Source: CAD feature listing. Evaluate the final solid. Frame: model axes, mm. Coordinates: 2 decimals unless noted, no trailing zeros. Loops run counter-clockwise (first coordinate to the right, second up) from the corner with the lowest first, then second, coordinate; pieces in that order, holes last. Notation, with made-up numbers: (-14, -32.5) - (22, -32.5) arc R29 ccw to (22, -0.5) - close; hole circle Ø2 at (19.5, 88). An arc over 180 degrees is marked (long way). Use one line per item in the form item = value. Start each with the question number.
from build123d import *

# Parameters (mm, degrees)
F0_R     = 11
F1_DEPTH = 1.5
F2_R     = 4
F3_DEPTH = 25


with BuildPart() as f1:
    # F0 (on Top) → F1 (new body)
    with BuildSketch(Plane.XY):
        with Locations((-33.321586, 31.793948)):
            Circle(F0_R)
    extrude(amount=F1_DEPTH)

    # F2 (on face) → F3 (cut)
    with BuildSketch(Plane.XY.offset(1.5)):
        with Locations((-33.321586, 31.793948)):
            Circle(F2_R)
    extrude(amount=-F3_DEPTH, mode=Mode.SUBTRACT)


with BuildPart() as f1_1:
    # F4: moved
    add(f1.part.moved(Location((22.4, -20.8, 0))))


solid = f1_1.part
(1) Mould query, pull axis Y, two halves, no side actions, for faces 1 (the face through (-14.096, 8.56, 0.76)), 2 (the face through (-5.01, 20.27, 0.74)), 3 (the face through (-11, 6, 0)). Classes: +Y half, -Y half, draft (parallel to the pull), parting line (faces both ways), or undercut.
(2) Cut plane B-B, the plane y = 10.5. Output: boundary loops of the cut face in (x, z).
(3) Contact query for a flat-ended pin moving along its axis: pin 1 (2 mm diameter, centred on x = -12, y = 18.5, fed in from -Z). Output: stop coordinate, or through.
(4) Cut plane D-D, the plane y = 16.5. Output: boundary loops of the cut face in (x, z).
(5) Material intervals for line 1 (X direction, y = 13.25, z = 0.2); line 2 (Y direction, x = -12.5, z = 1.25); line 3 (Y direction, x = -14, z = 1.25), sorted ascending.
(6) Cut plane C-C, the plane z = 1.2. Output: boundary loops of the cut face in (x, y), plus the area to 3 significant figures.
(7) Cut plane A-A, the plane x = -13.5. Output: boundary loops of the cut face in (y, z), plus the area to 3 significant figures.
Recorded:
q1.face_1 = undercut
q1.face_2 = parting line
q1.face_3 = draft
q2.outline = (-21.91, 0) - (-14.89, 0) - (-14.89, 1.5) - (-21.91, 1.5) - close; (-6.95, 0) - (0.07, 0) - (0.07, 1.5) - (-6.95, 1.5) - close
q3.pin_1 = 0
q4.outline = (-20.44, 0) - (-1.4, 0) - (-1.4, 1.5) - (-20.44, 1.5) - close
q5.line_1 = -21.69 to -14.22, -7.62 to -0.16
q5.line_2 = 0.11 to 7.32, 14.67 to 21.88
q5.line_3 = 0.43 to 8.44, 13.55 to 21.55
q6.outline = circle Ø22 at (-10.92, 10.99); hole circle Ø8 at (-10.92, 10.99)
q6.area = 330 mm²
q7.outline = (0.3, 0) - (7.94, 0) - (7.94, 1.5) - (0.3, 1.5) - close; (14.05, 0) - (21.69, 0) - (21.69, 1.5) - (14.05, 1.5) - close
q7.area = 22.9 mm²
